```python
from build123d import *

# Parameters (mm, degrees)
SALIENTE_EXTRUIR1_DEPTH = 15
CROQUIS3_R              = 17.5
SALIENTE_EXTRUIR2_DEPTH = 2
CROQUIS4_R              = 10
SALIENTE_EXTRUIR3_DEPTH = 3
CROQUIS6_R              = 0.75
CROQUIS7_R              = 5
SALIENTE_EXTRUIR4_DEPTH = 3
CROQUIS8_R              = 0.5
CORTAR_EXTRUIR2_DEPTH   = 39.213217609


with BuildPart() as part:
    # Croquis1 → Saliente-Extruir1 (new body)
    with BuildSketch(Plane(origin=(0, 0, 0), x_dir=(1, 0, 0), z_dir=(0, 1, 0))):
        Polygon((8.5, -13), (4.5, -4), (-4.5, -4), (-8.5, -13), (-12.5, -15), (-12.5, 0), (12.5, 0), (12.5, -15), align=None)
    extrude(amount=SALIENTE_EXTRUIR1_DEPTH)

    # Croquis3 → Saliente-Extruir2 (add)
    with BuildSketch(Plane(origin=(0, 0, 0), x_dir=(-1, 0, 0), z_dir=(0, 0, -1))):
        with Locations((0, 7.5)):
            Circle(CROQUIS3_R)
    extrude(amount=SALIENTE_EXTRUIR2_DEPTH)

    # Croquis4 → Saliente-Extruir3 (add)
    with BuildSketch(Plane(origin=(0, 0, -2), x_dir=(-1, 0, 0), z_dir=(0, 0, -1))):
        with Locations((0, 7.5)):
            Circle(CROQUIS4_R)
    extrude(amount=SALIENTE_EXTRUIR3_DEPTH)

    # Croquis6 → Cortar-Revolución1 (revolve, cut)
    with BuildSketch(Plane(origin=(0, 0, 0), x_dir=(0, 0, -1), z_dir=(1, 0, 0)), mode=Mode.PRIVATE) as cortar_revoluci_n1_sk:
        with Locations((3.5, 17.5)):
            Circle(CROQUIS6_R)
    revolve(cortar_revoluci_n1_sk.sketch.rotate(Axis((0, 7.5, -5), (0, 0, 1)), 90), axis=Axis((0, 7.5, -5), (0, 0, 1)), mode=Mode.SUBTRACT)

    # Croquis7 → Saliente-Extruir4 (add)
    with BuildSketch(Plane(origin=(0, 0, -5), x_dir=(-1, 0, 0), z_dir=(0, 0, -1))):
        with Locations((0, 7.5)):
            Circle(CROQUIS7_R)
    extrude(amount=SALIENTE_EXTRUIR4_DEPTH)

    # Croquis8 → Cortar-Extruir2 (cut, through all)
    with BuildSketch(Plane(origin=(0, 0, -8), x_dir=(-1, 0, 0), z_dir=(0, 0, -1))):
        with Locations((0, 7.5)):
            Circle(CROQUIS8_R)
    extrude(amount=-CORTAR_EXTRUIR2_DEPTH, mode=Mode.SUBTRACT)


solid = part.part
```
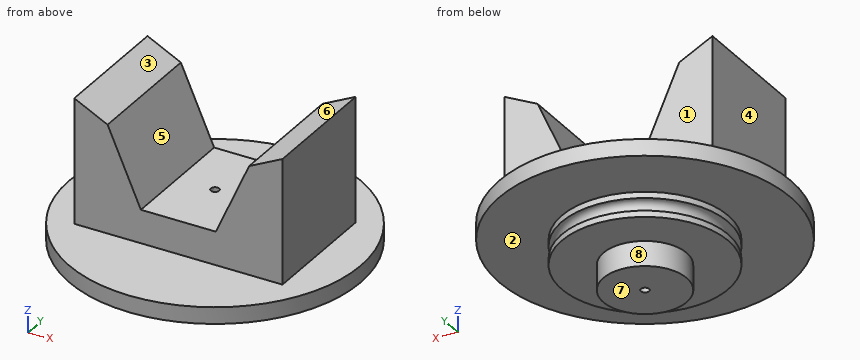
Model file for the job. Use its own axes, mm. Face numbers are marked on the shaded views. A direction names the side the tool comes from. Coordinates: 2 decimals unless noted, no trailing zeros. Order: outer loops, then holes, each group sorted by start corner. A loop starts at its lowest first (then second) coordinate and runs counter-clockwise, first axis right, second up. Notation, with made-up numbers: M 4,-14 L 9,-14 A14 ccw 9,-3 Z; hole C -17.5,-11.75 d2. An arc over 180 degrees is marked long. Answer as CSV lines item,"result".
(1) Band-saw the part on D-D, the plane z = -1.5. List the corners of the cut face in (x, y).
Geometry says:
outline,"C 0,7.5 d35; hole C 0,7.5 d1"
(2) Pull direction X, two halves, no side cores. Call the marked faces 5, 6, 7 and 8: +X half, -X half, draft (parallel to the pull), parting line (faces both ways), or undercut.
Geometry says:
face 5,"undercut"
face 6,"undercut"
face 7,"draft"
face 8,"parting line"
(3) Flat gauge pins, fed straight in: pin 1 (5 mm diameter, centred on x = 7, y = 11.5, fed in from -Z); pin 2 (12 mm diameter, centred on x = 10, y = 8.5, fed in from -Z); pin 3 (1.5 mm diameter, centred on x = -8, z = -4, fed in from +Y); pin 4 (7.5 mm diameter, centred on y = 5, z = 6, fed in from +X). Where does each tip first touch, or does it go through?
Geometry says:
pin 1,"stops at z = -5"
pin 2,"stops at z = -8"
pin 3,"stops at y = 14.34"
pin 4,"stops at x = 12.5"
(4) Band-saw the part on B-B, the plane y = 7.5. List the corners of the cut face in (x, z), then the cut area to 3 significant figures.
Geometry says:
outline,"M -17.5,-2 L -10,-2 L -10,-2.75 A0.75 cw -10,-4.25 L -10,-5 L -5,-5 L -5,-8 L -0.5,-8 L -0.5,4 L -4.5,4 L -8.5,13 L -12.5,15 L -12.5,0 L -17.5,0 Z; M 0.5,-8 L 5,-8 L 5,-5 L 10,-5 L 10,-4.25 A0.75 cw 10,-2.75 L 10,-2 L 17.5,-2 L 17.5,0 L 12.5,0 L 12.5,15 L 8.5,13 L 4.5,4 L 0.5,4 Z"
area,"362 mm2"
(5) Wall check: line 1 along Y through (x, z) = (0, -4.5); line 2 along Z through (x, y) = (-16, 1.5); line 3 along Y through (x, z) = (9, 9). Give the ranges that are in metal, low to high.
Geometry says:
line 1,"y = -2.5 to 7, 8 to 17.5"
line 2,"z = -2 to 0"
line 3,"y = 0 to 15"
(6) Band-saw the part on A-A, the plane x = 0. List the corners of the cut face in (y, z).
Geometry says:
outline,"M -10,-2 L -2.5,-2 L -2.5,-2.75 A0.75 cw -2.5,-4.25 L -2.5,-5 L 2.5,-5 L 2.5,-8 L 7,-8 L 7,4 L 0,4 L 0,0 L -10,0 Z; M 8,-8 L 12.5,-8 L 12.5,-5 L 17.5,-5 L 17.5,-4.25 A0.75 cw 17.5,-2.75 L 17.5,-2 L 25,-2 L 25,0 L 15,0 L 15,4 L 8,4 Z"
(7) 3-axis set-ups, long thin cutter, end or side, ignore diameter. For the marked faces 1, 2, 3 and 4: which of +Z, -Z, +X, -X, +Y, -Y reach the whole face in a straight line?
Geometry says:
face 1,"+Z, +X, -X, +Y"
face 2,"-Z"
face 3,"+Z, +Y, -Y"
face 4,"+Z, -X, +Y, -Y"
(8) Band-saw the part on C-C, the plane z = 8.25. List the corners of the cut face in (x, y), then the cut area to 3 significant figures.
Geometry says:
outline,"M -12.5,0 L -6.39,0 L -6.39,15 L -12.5,15 Z; M 6.39,0 L 12.5,0 L 12.5,15 L 6.39,15 Z"
area,"183 mm2"
